CAD build for the part. Positions are in the model's coordinates, mm. A direction names the side the tool comes from. Coordinates: 2 decimals unless noted, no trailing zeros. Write each loop counter-clockwise with the first axis right and the second up, starting at its lowest first coordinate (ties: lowest second). Pieces come first, ordered by that corner, then holes. Notation, with made-up numbers: (28.5, 42.25) - (35.5, 42.25) arc R9 ccw to (35.5, 48.25) - close; hole circle Ø1 at (-39, 23). An arc over 180 degrees is marked (long way). Answer in a Markdown table with one row per item. Add a question column.
Q1. Band-saw the part on A-A (y = 68.5). List the corners of the cut face in (x, z).
Q2. Band-saw the part on B-B (z = 134). List the corners of the cut face in (x, y), and give its area (3 significant figures).
Q3. Drill centre lines: line 1 along Z through (x, y) = (-9.5, -71.5); line 2 along X through (y, z) = (-77, 91.5); line 3 along X through (y, z) = (16.5, 88). Where is each one in solid material? Low to high. Write a range as from..to.
Q4. 3-axis set-ups, long thin cutter, end or side, ignore diameter. For faces 1 (the cylindrical face through (182.77, 1.75, 31.01)), 2 (the flat face through (-2, 2, 0)): which of +Z, -Z, +X, -X, +Y, -Y reach the whole face in a straight line?
Q5. Band-saw the part on D-D (x = -241). List the corners of the cut face in (y, z), and give its area (3 significant figures).
Q6. Two-plate mould, pull along X, no slides. Class faces 3 (the flat face through (-264.074, -1.75, 110.98)), 4 (the flat face through (245.703, -1.75, 119.16)), 5 (the flat face through (-292, -2, 180)): +X half, -X half, draft (parallel to the pull), parting line (faces both ways), or undercut.
Q7. Pin check, flat tips, straight feed: pin 1 (1.5 mm diameter, centred on x = -7, y = -78, fed in from +Z); pin 2 (10 mm diameter, centred on y = -17, z = 56, fed in from -X); pin 3 (4 mm diameter, centred on x = -227, y = -66, fed in from +Z). Stop position of each tip, or through.
Q8. Band-saw the part on C-C (x = 88). List the corners of the cut face in (y, z).
```python
from build123d import *

# Parameters (mm, degrees)
F0_W     = 400
F0_H     = 250
F1_DEPTH = 20
F3_DEPTH = 250
F4_R     = 80


# Not quite as in the source:
# - a pattern or mirror of a feature is missing from the dataset's text; its kind, count and spacing are read off the source's solid


with BuildPart() as f1:
    # F0 (on Top) → F1 (new body)
    with BuildSketch(Plane.XY):
        Rectangle(F0_W, F0_H)
    extrude(amount=F1_DEPTH)

    # F2 (on face) → F3 (join, through all)
    with BuildSketch(Plane.XZ.offset(125)):
        Polygon((-303.9230484541, 180), (-200, 0), (-188.4529946162, 20), (-280.8290376865, 180), align=None)
    f3 = extrude(amount=-F3_DEPTH)

    # F3_copies: F3 across plane
    add(f3.mirror(Plane(origin=(0, 0, 0), x_dir=(0, 0, 1), z_dir=(1, 0, 0))))

    # F4
    f4_edges = [f1.edges().sort_by_distance(p)[0] for p in [
        (-188.452995, 0, 20),
        (-200, 0, 0),
        (188.452995, 0, 20),
        (200, 0, 0),
    ]]
    fillet(f4_edges, radius=F4_R)


solid = f1.part
```
Checked values:
| question | item | result |
|---|---|---|
| 1 | outline | (-303.92, 180) - (-223.09, 40) arc R80 ccw to (-153.81, 0) - (153.81, 0) arc R80 ccw to (223.09, 40) - (303.92, 180) - (280.83, 180) - (211.55, 60) arc R80 cw to (142.26, 20) - (-142.26, 20) arc R80 cw to (-211.55, 60) - (-280.83, 180) - close |
| 2 | outline | (-277.36, -125) - (-254.27, -125) - (-254.27, 125) - (-277.36, 125) - close; (254.27, -125) - (277.36, -125) - (277.36, 125) - (254.27, 125) - close |
| 2 | area | 11,500 mm² |
| 3 | line 1 | z = 0..20 |
| 3 | line 2 | x = -252.83..-229.73, 229.73..252.83 |
| 3 | line 3 | x = -250.81..-227.71, 227.71..250.81 |
| 4 | face 1 | +Z, +Y, -Y |
| 4 | face 2 | -Z, +X, -X, +Y, -Y |
| 5 | outline | (-125, 71.01) - (125, 71.01) - (125, 111.01) - (-125, 111.01) - close |
| 5 | area | 10,000 mm² |
| 6 | face 3 | -X half |
| 6 | face 4 | undercut |
| 6 | face 5 | draft |
| 7 | pin 1 | stops at z = 20 |
| 7 | pin 2 | stops at x = -235.22 |
| 7 | pin 3 | stops at z = 90.23 |
| 8 | outline | (-125, 0) - (125, 0) - (125, 20) - (-125, 20) - close |
